Autodesk Inventor part; units mm, degrees
ref_plane "YZ Plane" through (0, 0, 0) normal (1, 0, 0) x (0, 1, 0)
ref_plane "XZ Plane" through (0, 0, 0) normal (0, 1, 0) x (-1, 0, 0)
ref_plane "XY Plane" through (0, 0, 0) normal (0, 0, 1) x (1, 0, 0)
sketch "Эскиз1" plane through (0, 0, 0) normal (0, 0, 1) x (1, 0, 0)
  line L0 (0, 0) -> (0, 595)
  line L1 (5, 600) -> (147, 600)
  line L2 (153, 600) -> (298.5355, 454.4645)
  line L3 (300, 450.9289) -> (300, 0)
  line L4 (300, 0) -> (281.25, 0)
  line L5 (281.25, 0) -> (281.25, -6)
  line L6 (281.25, -6) -> (243.75, -6)
  line L7 (243.75, -6) -> (243.75, 0)
  line L8 (243.75, 0) -> (206.25, 0)
  line L9 (206.25, 0) -> (206.25, -6)
  line L10 (206.25, -6) -> (168.75, -6)
  line L11 (168.75, -6) -> (168.75, 0)
  line L12 (168.75, 0) -> (131.25, 0)
  line L13 (131.25, 0) -> (131.25, -6)
  line L14 (131.25, -6) -> (93.75, -6)
  line L15 (93.75, -6) -> (93.75, 0)
  line L16 (93.75, 0) -> (56.25, 0)
  line L17 (56.25, 0) -> (56.25, -6)
  line L18 (56.25, -6) -> (18.75, -6)
  line L19 (18.75, -6) -> (18.75, 0)
  line L20 (18.75, 0) -> (0, 0)
  line L21 (18.75, 0) -> (-18.75, 0) construction
  line L22 (281.25, 0) -> (318.75, 0) construction
  line L23 (153, 600) -> (147, 600) construction
  line L24 (150, 600) -> (150, 0) construction
  line L25 (0, 300) -> (150, 300) construction
  line L26 (150, 300) -> (300, 300) construction
  arc A0 (37.5, 375) -> (37.5, 360) centre (37.5, 367.5) ccw
  line L27 (37.5, 360) -> (112.5, 360)
  line L28 (37.5, 375) -> (112.5, 375)
  line L29 (75, 375) -> (75, 360) construction
  arc A1 (112.5, 360) -> (112.5, 375) centre (112.5, 367.5) ccw
  line L30 (37.5, 367.5) -> (0, 367.5) construction
  line L31 (112.5, 367.5) -> (150, 367.5) construction
  line L32 (37.5, 300) -> (112.5, 300)
  arc A2 (112.5, 300) -> (112.5, 315) centre (112.5, 307.5) ccw
  line L33 (37.5, 315) -> (112.5, 315)
  arc A3 (37.5, 315) -> (37.5, 300) centre (37.5, 307.5) ccw
  line L34 (37.5, 240) -> (112.5, 240)
  arc A4 (112.5, 240) -> (112.5, 255) centre (112.5, 247.5) ccw
  line L35 (37.5, 255) -> (112.5, 255)
  arc A5 (37.5, 255) -> (37.5, 240) centre (37.5, 247.5) ccw
  line L36 (37.5, 180) -> (112.5, 180)
  arc A6 (112.5, 180) -> (112.5, 195) centre (112.5, 187.5) ccw
  line L37 (37.5, 195) -> (112.5, 195)
  arc A7 (37.5, 195) -> (37.5, 180) centre (37.5, 187.5) ccw
  line L38 (37.5, 120) -> (112.5, 120)
  arc A8 (112.5, 120) -> (112.5, 135) centre (112.5, 127.5) ccw
  line L39 (37.5, 135) -> (112.5, 135)
  arc A9 (37.5, 135) -> (37.5, 120) centre (37.5, 127.5) ccw
  line L40 (37.5, 60) -> (112.5, 60)
  arc A10 (112.5, 60) -> (112.5, 75) centre (112.5, 67.5) ccw
  line L41 (37.5, 75) -> (112.5, 75)
  arc A11 (37.5, 75) -> (37.5, 60) centre (37.5, 67.5) ccw
  line L42 (153, 300) -> (147, 300)
  line L43 (153, 300) -> (153, 600)
  line L44 (147, 300) -> (147, 600)
  arc A12 (300, 450.9289) -> (298.5355, 454.4645) centre (295, 450.9289) ccw
  arc A13 (5, 600) -> (0, 595) centre (5, 595) ccw
  point P0 (0, 600)
  point P1 (300, 453)
  point P2 (75, 300)
  point P3 (75, 315)
  point P4 (75, 240)
  point P5 (75, 255)
  point P6 (75, 180)
  point P7 (75, 195)
  point P8 (75, 120)
  point P9 (75, 135)
  point P10 (75, 60)
  point P11 (75, 75)
  dimension "d0" = 6
  dimension "d1" = 300
  dimension "d3" = 135
  dimension "d4" = 153
  dimension "d7" = 15
  dimension "d8" = 75
  dimension "d9" = 225
  dimension "d12" = 60
  dimension "d17" = 6
  dimension "d18" = 5
  dimension "d19" = 5
  dimension "d20" = 600
extrude "Корпус" add sketch "Эскиз1" along normal blind 6
sketch "Эскиз2" plane through (0, 0, 0) normal (0, 0, -1) x (-1, 0, 0)
  line L0 (-227, -6) -> (-227, 0) construction
  line L1 (-223, -6) -> (-223, 0) construction
  line L2 (-227, 0) -> (-227, 5.95)
  line L3 (-227, 5.95) -> (-228.4, 5.95)
  line L4 (-228.4, 5.95) -> (-228.4, 9.05)
  line L5 (-228.4, 9.05) -> (-227, 9.05)
  line L6 (-227, 9.05) -> (-227, 15)
  line L7 (-227, 15) -> (-223, 15)
  line L8 (-223, 15) -> (-223, 9.05)
  line L9 (-223, 9.05) -> (-221.6, 9.05)
  line L10 (-221.6, 9.05) -> (-221.6, 5.95)
  line L11 (-221.6, 5.95) -> (-223, 5.95)
  line L12 (-223, 5.95) -> (-223, 0)
  line L13 (-153, 55) -> (-153, 595) construction
  line L14 (-147, 55) -> (-147, 595) construction
  line L15 (-153, 595) -> (-147, 595) construction
  line L16 (-153, 55) -> (-147, 55) construction
  line L17 (-150, 595) -> (-150, 55) construction
  line L18 (-227, 0) -> (-223, 0)
  line L19 (-73, 0) -> (-73, 5.95)
  line L20 (-73, 5.95) -> (-71.6, 5.95)
  line L21 (-71.6, 5.95) -> (-71.6, 9.05)
  line L22 (-71.6, 9.05) -> (-73, 9.05)
  line L23 (-73, 9.05) -> (-73, 15)
  line L24 (-73, 15) -> (-77, 15)
  line L25 (-77, 15) -> (-77, 9.05)
  line L26 (-77, 9.05) -> (-78.4, 9.05)
  line L27 (-78.4, 9.05) -> (-78.4, 5.95)
  line L28 (-78.4, 5.95) -> (-77, 5.95)
  line L29 (-77, 5.95) -> (-77, 0)
  line L30 (-73, 0) -> (-77, 0)
  point P0 (0, 0)
  dimension "d21" = 15
  dimension "d22" = 3.1
  dimension "d23" = 6.8
extrude "Пазы" cut sketch "Эскиз2" against normal blind 6
equation "\"d8\" = 0.25 * d1"
equation "\"d9\" = 15 * d7"
equation "\"d12\" = 4 * d7"
equation "\"d17\" = d0"
equation "\"d5\" = d0"
equation "\"d24\" = d0"
properties part number "Korpus"
Work out the finished part from the listing and answer in its coordinate system (mm). Coordinates: 2 decimals unless noted, no trailing zeros. Write each loop counter-clockwise with the first axis right and the second up, starting at its lowest first coordinate (ties: lowest second). Pieces come first, ordered by that corner, then holes.
Q1. A cutting plane is placed at C-C, the plane y = 307.5. Give the vertices of the cut face in (x, z).
Q2. A cutting plane is placed at A-A, the plane y = 554.5. Give the vertices of the cut face in (x, z), then the cut area to 4 significant figures.
Q3. A cutting plane is placed at B-B, the plane x = 46.5. Give the vertices of the cut face in (y, z), then the cut area to 3 significant figures.
Q4. Find the intervals of material crossed by line 1 (X direction, y = 436.5, z = 2.85); line 2 (Y direction, x = 132.5, z = 3.15); line 3 (X direction, y = 508, z = 0.5), in increasing order.
Q5. Each of these flat-tipped pins is pushed along its axis until it touches: pin 1 Ø3 at (x, z) = (288.5, 4.5) entering from -Y; pin 2 Ø1.8 at (y, z) = (-4, 3.5) entering from +X. Where does it stop, or does it pass through?
Q6. A cutting plane is placed at D-D, the plane y = 187.5. Give the vertices of the cut face in (x, z), then the cut area to 3 significant figures.
Findings below:
1. outline: (0, 0) - (30, 0) - (30, 6) - (0, 6) - close; (120, 0) - (147, 0) - (147, 6) - (120, 6) - close; (153, 0) - (300, 0) - (300, 6) - (153, 6) - close
2. outline: (0, 0) - (147, 0) - (147, 6) - (0, 6) - close; (153, 0) - (198.5, 0) - (198.5, 6) - (153, 6) - close
2. area: 1,155 mm2
3. outline: (-6, 0) - (60, 0) - (60, 6) - (-6, 6) - close; (75, 0) - (120, 0) - (120, 6) - (75, 6) - close; (135, 0) - (180, 0) - (180, 6) - (135, 6) - close; (195, 0) - (240, 0) - (240, 6) - (195, 6) - close; (255, 0) - (300, 0) - (300, 6) - (255, 6) - close; (315, 0) - (360, 0) - (360, 6) - (315, 6) - close; (375, 0) - (600, 0) - (600, 6) - (375, 6) - close
3. area: 3,100 mm2
4. line 1: x = 0 to 147, 153 to 300
4. line 2: y = 0 to 600
4. line 3: x = 0 to 147, 153 to 245
5. pin 1: stops at y = 0
5. pin 2: stops at x = 281.25
6. outline: (0, 0) - (30, 0) - (30, 6) - (0, 6) - close; (120, 0) - (300, 0) - (300, 6) - (120, 6) - close
6. area: 1,260 mm2
